from build123d import *

# Parameters (mm, degrees)
ESQUISSE1_W             = 35
ESQUISSE1_H             = 40
BOSS_EXTRU_1_DEPTH      = 3
ESQUISSE2_R             = 2.013179567
ESQUISSE2_R_2           = 1.5
ENL_V_MAT_EXTRU_1_DEPTH = 10
ESQUISSE3_W             = 35
ESQUISSE3_H             = 3
BOSS_EXTRU_2_DEPTH      = 5
ESQUISSE4_W             = 4
ESQUISSE4_H             = 45
ESQUISSE4_W_2           = 12.966129595
ESQUISSE4_H_2           = 5
BOSS_EXTRU_3_DEPTH      = 15
BOSS_EXTRU_4_DEPTH      = 10
ESQUISSE6_W             = 5
ESQUISSE6_H             = 5.175
BOSS_EXTRU_5_DEPTH      = 15
ESQUISSE7_W             = 18
ESQUISSE7_H             = 55
BOSS_EXTRU_6_DEPTH      = 3
BOSS_EXTRU_7_DEPTH      = 3
BOSS_EXTRU_8_DEPTH      = 3
ESQUISSE10_R            = 1.25
ENL_V_MAT_EXTRU_2_DEPTH = 6
ESQUISSE11_W            = 5
ESQUISSE11_H            = 8
BOSS_EXTRU_9_DEPTH      = 8
ESQUISSE12_R            = 1.4
ENL_V_MAT_EXTRU_3_DEPTH = 8
ESQUISSE13_W            = 7.966129595
ESQUISSE13_H            = 8.175
BOSS_EXTRU_10_DEPTH     = 2
BOSS_EXTRU_12_START     = 2
ESQUISSE14_W            = 12
ESQUISSE14_H            = 5
ESQUISSE14_R            = 1.5
BOSS_EXTRU_12_DEPTH     = 2
CONG_1_R                = 3
ENL_V_START             = -2
ESQUISSE15_R            = 3.5
ESQUISSE15_R_2          = 1.5
ENL_V_MAT_EXTRU_4_DEPTH = 2


with BuildPart() as part:
    # Esquisse1 → Boss.-Extru.1 (new body)
    with BuildSketch(Plane.XY):
        Rectangle(ESQUISSE1_W, ESQUISSE1_H)
    extrude(amount=BOSS_EXTRU_1_DEPTH)

    # Esquisse2 → Enlèv. mat.-Extru.1 (cut)
    with BuildSketch(Plane.XY.offset(3)):
        with Locations((-7.5, 634.376711736)):
            Circle(ESQUISSE2_R)
        with Locations((-7.023580812, 615.376711736)):
            Circle(ESQUISSE2_R)
        with Locations((-7.5, 2.5)):
            Circle(ESQUISSE2_R_2)
        with Locations((-7.5, -16.5)):
            Circle(ESQUISSE2_R_2)
    extrude(amount=-ENL_V_MAT_EXTRU_1_DEPTH, mode=Mode.SUBTRACT)

    # Esquisse3 → Boss.-Extru.2 (add)
    with BuildSketch(Plane.XZ.offset(20)):
        with Locations((0, 1.5)):
            Rectangle(ESQUISSE3_W, ESQUISSE3_H)
    extrude(amount=BOSS_EXTRU_2_DEPTH)

    # Esquisse4 → Boss.-Extru.3 (add)
    with BuildSketch(Plane.XY.offset(3)):
        with Locations((15.5, -2.5)):
            Rectangle(ESQUISSE4_W, ESQUISSE4_H)
        with Locations((-11.016935203, -22.5)):
            Rectangle(ESQUISSE4_W_2, ESQUISSE4_H_2)
    extrude(amount=BOSS_EXTRU_3_DEPTH)

    # Esquisse5 → Boss.-Extru.4 (add)
    with BuildSketch(Plane(origin=(0, 20, 0), x_dir=(1, 0, 0), z_dir=(0, 1, 0))):
        Polygon((17.5, 0), (-17.5, 0), (-17.5, -3), (13.5, -3), (13.5, -18), (17.5, -18), align=None)
    extrude(amount=BOSS_EXTRU_4_DEPTH)

    # Esquisse6 → Boss.-Extru.5 (add)
    with BuildSketch(Plane.XY.offset(3)):
        with Locations((-7.033870405, 27.4125)):
            Rectangle(ESQUISSE6_W, ESQUISSE6_H)
    extrude(amount=BOSS_EXTRU_5_DEPTH)

    # Esquisse7 → Boss.-Extru.6 (add)
    with BuildSketch(Plane(origin=(17.5, 0, 0), x_dir=(0, 0, -1), z_dir=(1, 0, 0))):
        with Locations((-9, 2.5)):
            Rectangle(ESQUISSE7_W, ESQUISSE7_H)
    extrude(amount=BOSS_EXTRU_6_DEPTH)

    # Esquisse8 → Boss.-Extru.7 (add)
    with BuildSketch(Plane.XZ.offset(25)):
        Polygon((-17.5, 18), (-17.5, 0), (20.5, 0), (20.5, 18), (13.5, 18), (13.5, 3), (-4.533870405, 3), (-4.533870405, 18), align=None)
    extrude(amount=BOSS_EXTRU_7_DEPTH)

    # Esquisse9 → Boss.-Extru.8 (add)
    with BuildSketch(Plane(origin=(0, 30, 0), x_dir=(1, 0, 0), z_dir=(0, 1, 0))):
        Polygon((13.5, -18), (20.5, -18), (20.5, 0), (-17.5, 0), (-17.5, -3), (-9.533870405, -3), (-9.533870405, -18), (-4.533870405, -18), (-4.533870405, -3), (13.5, -3), align=None)
    extrude(amount=BOSS_EXTRU_8_DEPTH)

    # Esquisse10 → Enlèv. mat.-Extru.2 (cut)
    with BuildSketch(Plane.XY.offset(18)):
        with Locations((17, -23)):
            Circle(ESQUISSE10_R)
        with Locations((17, 28)):
            Circle(ESQUISSE10_R)
        with Locations((-11.016935202, -24)):
            Circle(ESQUISSE10_R)
        with Locations((-7.033870405, 28)):
            Circle(ESQUISSE10_R)
    extrude(amount=-ENL_V_MAT_EXTRU_2_DEPTH, mode=Mode.SUBTRACT)

    # Esquisse11 → Boss.-Extru.9 (add)
    with BuildSketch(Plane(origin=(20.5, 0, 0), x_dir=(0, 0, -1), z_dir=(1, 0, 0))):
        with Locations((-2.5, -24)):
            Rectangle(ESQUISSE11_W, ESQUISSE11_H)
        with Locations((-2.5, 29)):
            Rectangle(ESQUISSE11_W, ESQUISSE11_H)
    boss_extru_9 = extrude(amount=BOSS_EXTRU_9_DEPTH)

    # Esquisse12 → Enlèv. mat.-Extru.3 (cut)
    with BuildSketch(Plane.XY.offset(5)):
        with Locations((24.5, -24)):
            Circle(ESQUISSE12_R)
        with Locations(Location((24.5, 29, 0), (0, 0, 180))):
            Circle(ESQUISSE12_R)
    enl_v_mat_extru_3 = extrude(amount=-ENL_V_MAT_EXTRU_3_DEPTH, mode=Mode.SUBTRACT)

    # Symétrie1: Boss.-Extru.9, Enlèv. mat.-Extru.3 across plane
    add(boss_extru_9.mirror(Plane(origin=(1.5, 0, 0), x_dir=(0, 0, 1), z_dir=(1, 0, 0))))
    add(enl_v_mat_extru_3.mirror(Plane(origin=(1.5, 0, 0), x_dir=(0, 0, 1), z_dir=(1, 0, 0))), mode=Mode.SUBTRACT)

    # Esquisse13 → Boss.-Extru.10 (add)
    with BuildSketch(Plane.XY.offset(3)):
        with Locations((-13.516935203, 28.9125)):
            Rectangle(ESQUISSE13_W, ESQUISSE13_H)
    extrude(amount=BOSS_EXTRU_10_DEPTH)

    # Esquisse14 → Boss.-Extru.12 (add)
    # profile 1 of 3: a face of its own
    with BuildSketch(Plane.XY.offset(3).offset(BOSS_EXTRU_12_START)):
        with Locations((-11.5, 17.325)):
            Rectangle(ESQUISSE14_W, ESQUISSE14_H)
    # profile 2 of 3: a face of its own
    with BuildSketch(Plane.XY.offset(3).offset(BOSS_EXTRU_12_START)):
        with Locations((-11.5, 2.5)):
            Rectangle(ESQUISSE14_W, ESQUISSE14_H)
        with Locations((-7.5, 2.5)):
            Circle(ESQUISSE14_R, mode=Mode.SUBTRACT)
    # profile 3 of 3: a face of its own
    with BuildSketch(Plane.XY.offset(3).offset(BOSS_EXTRU_12_START)):
        with Locations((-11.5, -16.5)):
            Rectangle(ESQUISSE14_W, ESQUISSE14_H)
        with Locations((-7.5, -16.5)):
            Circle(ESQUISSE14_R, mode=Mode.SUBTRACT)
    extrude(amount=-BOSS_EXTRU_12_DEPTH)

    # Congé1
    cong_1_edges = [part.edges().sort_by_distance(p)[0] for p in [
        (-25.5, 33, 2.5),
        (-25.5, 25, 2.5),
        (-25.5, -28, 2.5),
        (-25.5, -20, 2.5),
        (28.5, 33, 2.5),
        (28.5, 25, 2.5),
        (28.5, -20, 2.5),
        (28.5, -28, 2.5),
    ]]
    fillet(cong_1_edges, radius=CONG_1_R)

    # Esquisse15 → Enlèv. mat.-Extru.4 (cut)
    # profile 1 of 2: a face of its own
    with BuildSketch(Plane(origin=(0, 0, 0), x_dir=(-1, 0, 0), z_dir=(0, 0, -1)).offset(ENL_V_START)):
        with Locations((7.5, 2.5)):
            Circle(ESQUISSE15_R)
        with Locations(Location((7.5, 2.5, 0), (0, 0, 180))):
            Circle(ESQUISSE15_R_2, mode=Mode.SUBTRACT)
    # profile 2 of 2: a face of its own
    with BuildSketch(Plane(origin=(0, 0, 0), x_dir=(-1, 0, 0), z_dir=(0, 0, -1)).offset(ENL_V_START)):
        with Locations((7.5, -16.5)):
            Circle(ESQUISSE15_R)
        with Locations(Location((7.5, -16.5, 0), (0, 0, 180))):
            Circle(ESQUISSE15_R_2, mode=Mode.SUBTRACT)
    extrude(amount=ENL_V_MAT_EXTRU_4_DEPTH, mode=Mode.SUBTRACT)


solid = part.part
Read the model definition and answer for the solid it produces. Units are mm, in the model's axes. A direction names the side the tool comes from. Coordinates: 2 decimals unless noted, no trailing zeros. Write each loop counter-clockwise with the first axis right and the second up, starting at its lowest first coordinate (ties: lowest second). Pieces come first, ordered by that corner, then holes. Notation, with made-up numbers: M -2,48.5 L 7,48.5 A22 ccw 7,77.5 Z; hole C 78,-2 d11. An arc over 180 degrees is marked long. Use a Markdown table: item, result.
Q1. The part is cut by section B-B, the plane x = 24.5. Write down the section's boundary in (y, z), then the cut area to 3 significant figures.
Answer block:
| item | result |
|---|---|
| outline | M -28,0 L -25.4,0 L -25.4,5 L -28,5 Z; M -22.6,0 L -20,0 L -20,5 L -22.6,5 Z; M 25,0 L 27.6,0 L 27.6,5 L 25,5 Z; M 30.4,0 L 33,0 L 33,5 L 30.4,5 Z |
| area | 52.0 mm2 |
Q2. Straight lines are drawn through the part: L1, parallel to Y at x = -5, z = 17 (3 decimals); L2, parallel to X at y = 29.5, z = 7.75; L3, parallel to Y at x = -21.5, z = 2.35. For each, find the intervals that lie inside material, in ascending order. Write a range as [from, to].
Answer block:
| item | result |
|---|---|
| L1 | y = [-28, -20], [24.825, 33] |
| L2 | x = [-9.53, -4.53], [13.5, 20.5] |
| L3 | y = [-28, -25.4], [-22.6, -20], [25, 27.6], [30.4, 33] |
Q3. Determine the mould class of faces 1 (the face through (-22.15, -25.24, 2.54)), 2 (the face through (1, 33, 1)), 3 (the face through (13.5, 2, 10)) for opening direction Y: released by +Y, released by -Y, zero draft, split by the parting line, or undercut.
Answer block:
| item | result |
|---|---|
| face 1 | undercut |
| face 2 | released by +Y |
| face 3 | zero draft |
Q4. Each of these flat-tipped pins is pushed along its axis until it touches: pin 1 Ø6.5 at (x, y) = (-7.5, 2.5) entering from -Z; pin 2 Ø2.5 at (x, y) = (-10, -16) entering from +Z; pin 3 Ø2 at (y, z) = (-16, 4.5) entering from +X; pin 4 Ø1 at (x, z) = (-18.5, 11.5) entering from +Y. Where does it stop, or does it pass through?
Answer block:
| item | result |
|---|---|
| pin 1 | stops at z = 2 |
| pin 2 | stops at z = 5 |
| pin 3 | stops at x = 20.5 |
| pin 4 | passes through |
Q5. The part is cut by section C-C, the plane z = 10.25. Write down the section's boundary in (x, y) (3 decimals), then the cut area to 3 significant figures.
Answer block:
| item | result |
|---|---|
| outline | M -17.5,-28 L -4.534,-28 L -4.534,-20 L -17.5,-20 Z; M -9.534,24.825 L -4.534,24.825 L -4.534,33 L -9.534,33 Z; M 13.5,-28 L 20.5,-28 L 20.5,33 L 13.5,33 Z |
| area | 572 mm2 |
Q6. Which of the six approach directions +Z, -Z, +X, -X, +Y, -Y give full straight-line access (tool end or side, diameter ignored) to faces 4 (the face through (-17.5, -24, 11)), 5 (the face through (-24.64, -20.9, 2.46)), 6 (the face through (16.73, -24.22, 15.04)), 7 (the face through (-11, -20, 9))?
Answer block:
| item | result |
|---|---|
| face 4 | +Z, -X, +Y, -Y |
| face 5 | +Z, -Z, -X |
| face 6 | +Z |
| face 7 | +Z, -X |
Q7. The part is cut by section D-D, the plane y = 18. Write down the section's boundary in (x, z).
Answer block:
| item | result |
|---|---|
| outline | M -17.5,0 L 20.5,0 L 20.5,18 L 13.5,18 L 13.5,3 L -5.5,3 L -5.5,5 L -17.5,5 Z |
Q8. The part is cut by section A-A, the plane z = 16.75. Write down the section's boundary in (x, y) (3 decimals).
Answer block:
| item | result |
|---|---|
| outline | M -17.5,-28 L -4.534,-28 L -4.534,-20 L -17.5,-20 Z; M -9.534,24.825 L -4.534,24.825 L -4.534,33 L -9.534,33 Z; M 13.5,-28 L 20.5,-28 L 20.5,33 L 13.5,33 Z; hole C -11.017,-24 d2.5; hole C -7.034,28 d2.5; hole C 17,-23 d2.5; hole C 17,28 d2.5 |
